Print and shaded views of the part. All mm, measured from the part's lowest x, y and z. Coordinates: 2 decimals unless noted, no trailing zeros. Order: outer loops, then holes, each group sorted by start corner. A loop starts at its lowest first (then second) coordinate and runs counter-clockwise, first axis right, second up. Notation, with made-up numbers: M -26,-4.75 L -17,-4.75 A37 cw -17,32.25 Z; hole C 66.25,62 d6. An arc over 180 degrees is marked long. Return JSON: item names as keys, results as strings.
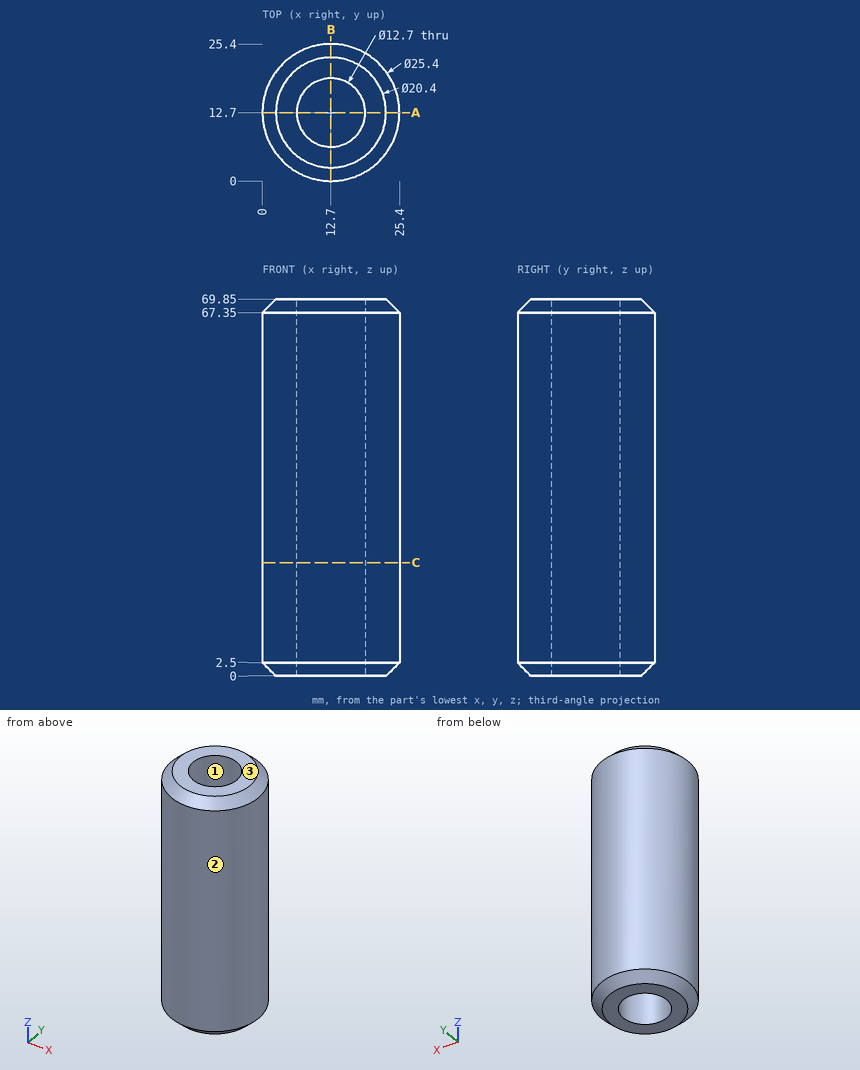
Item 1: Saw through at A-A (y = 12.7). Write the cut outline in (x, z), and give its area (3 significant figures).
Check result:
{"outline": "M 0,2.5 L 2.5,0 L 6.35,0 L 6.35,69.85 L 2.5,69.85 L 0,67.35 Z; M 19.05,0 L 22.9,0 L 25.4,2.5 L 25.4,67.35 L 22.9,69.85 L 19.05,69.85 Z", "area": "875 mm2"}
Item 2: Drop flat-ended pins along their axis: pin 1 Ø6 at (x, z) = (19, 44.5) entering from +Y; pin 2 Ø1.5 at (y, z) = (9, 55) entering from +X; pin 3 Ø5 at (y, z) = (4, 36.5) entering from -X. Give the stop position or say it passes through.
Check result:
{"pin 1": "stops at y = 24.96", "pin 2": "stops at x = 25.05", "pin 3": "stops at x = 1.62"}
Item 3: Pull direction Y, two halves, no side cores. Call the marked faces 1, 2 and 3: +Y half, -Y half, draft (parallel to the pull), parting line (faces both ways), or undercut.
Check result:
{"face 1": "undercut", "face 2": "parting line", "face 3": "draft"}
Item 4: Wall check: line 1 (Y direction, x = 12.7, z = 41); line 2 (Y direction, x = 8.75, z = 44); line 3 (X direction, y = 11.75, z = 28). Give the ranges that are in metal, low to high.
Check result:
{"line 1": "y = 0 to 6.35, 19.05 to 25.4", "line 2": "y = 0.63 to 7.73, 17.67 to 24.77", "line 3": "x = 0.04 to 6.42, 18.98 to 25.36"}
Item 5: Saw through at C-C (z = 21). Write the cut outline in (x, y).
Check result:
{"outline": "C 12.7,12.7 d25.4; hole C 12.7,12.7 d12.7"}
